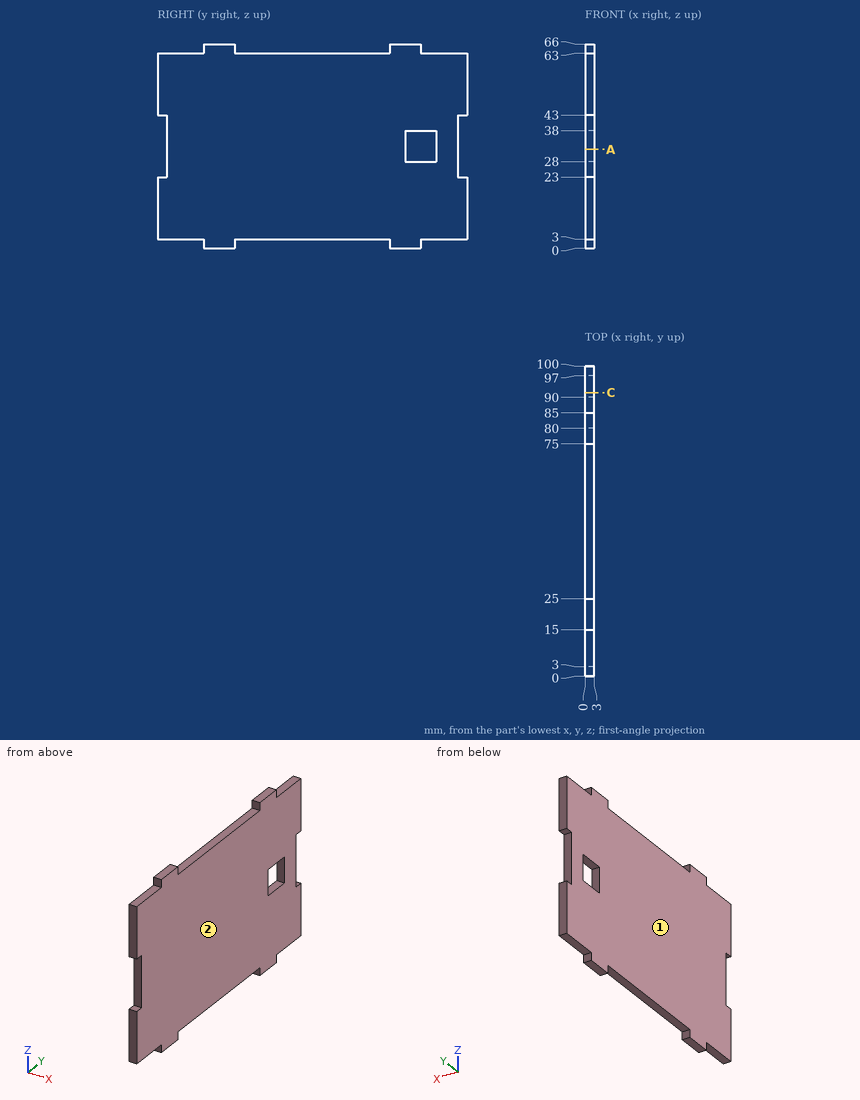
Geometry: see drawing. Coordinates: mm, zero at the bounding-box minimum. Round coordinates to 2 decimals unless told otherwise and drop trailing zeros. Loops run counter-clockwise (first coordinate to the right, second up) from the corner with the lowest first, then second, coordinate; pieces in that order, holes last. Notation, with made-up numbers: M 48.5,66 L 72.5,66 A20 ccw 72.5,74 Z; hole C 51,60 d10. An arc over 180 degrees is marked long. Use a Markdown table: item, result. Add a question column.
1. Pull-direction query (X, two-part tool) for the marked faces 1 and 2; classes: +X half, -X half, draft (parallel to the pull), parting line (faces both ways), or undercut.
2. Ray query, line 1 along Y through (x, z) = (1.8, 33.5); line 2 along Z through (x, y) = (0.9, 83.5); line 3 along Z through (x, y) = (1.8, 90.5). Return the intervals inside material, ascending. Write a range as [from, to].
3. Cut plane C-C, the plane y = 91.5. Output: boundary loops of the cut face in (x, z), and give its area (3 significant figures).
4. Contact query for flat-ended pins moving along their axis: pin 1 (1.5 mm diameter, centred on x = 1.5, z = 1, fed in from +Y); pin 2 (0.9 mm diameter, centred on x = 1.5, z = 1, fed in from -Y); pin 3 (0.9 mm diameter, centred on x = 1, z = 29.5, fed in from -Y). Output: stop coordinate, or through.
5. Cut plane A-A, the plane z = 32. Output: boundary loops of the cut face in (x, y), and give its area (3 significant figures).
Solution:
| question | item | result |
|---|---|---|
| 1 | face 1 | -X half |
| 1 | face 2 | +X half |
| 2 | line 1 | y = [3, 80], [90, 97] |
| 2 | line 2 | z = [0, 28], [38, 66] |
| 2 | line 3 | z = [3, 63] |
| 3 | outline | M 0,3 L 3,3 L 3,63 L 0,63 Z |
| 3 | area | 180 mm2 |
| 4 | pin 1 | stops at y = 85 |
| 4 | pin 2 | stops at y = 15 |
| 4 | pin 3 | stops at y = 3 |
| 5 | outline | M 0,3 L 3,3 L 3,80 L 0,80 Z; M 0,90 L 3,90 L 3,97 L 0,97 Z |
| 5 | area | 252 mm2 |
